```python
from build123d import *

# Parameters (mm, degrees)
EXTRUDE_1_DEPTH     = 50
SKETCH_3_R          = 2.5
CUT_EXTRUDE_1_DEPTH = 74.539294107
SKETCH_4_W          = 29.863739494
SKETCH_4_H          = 8.563866473
EXTRUDE_2_DEPTH     = 37


with BuildPart() as part:
    # 草图2 → 凸台-拉伸1 (new, symmetric)
    with BuildSketch(Plane.XY):
        Polygon((-30, 19.5), (30, 19.5), (30, -16.666666667), (40, -16.666666667), (40, -19.5), (-40, -19.5), (-40, -16.666666667), (-30, -16.666666667), align=None)
    extrude(amount=EXTRUDE_1_DEPTH, both=True)

    # 草图3 → 切除-拉伸1 (cut, through all)
    with BuildSketch(Plane(origin=(0, -16.666666667, 0), x_dir=(1, 0, 0), z_dir=(0, 1, 0))):
        with Locations(Location((-35, 24, 0), (0, 0, 270))):
            Circle(SKETCH_3_R)
        with Locations(Location((35, 24, 0), (0, 0, 270))):
            Circle(SKETCH_3_R)
        with Locations(Location((-35, -24, 0), (0, 0, 270))):
            Circle(SKETCH_3_R)
        with Locations(Location((35, -24, 0), (0, 0, 270))):
            Circle(SKETCH_3_R)
    extrude(amount=-CUT_EXTRUDE_1_DEPTH, mode=Mode.SUBTRACT)

    # 草图4 → 凸台-拉伸2 (add)
    with BuildSketch(Plane.XY.offset(50)):
        with Locations((0, -12.959263215)):
            Rectangle(SKETCH_4_W, SKETCH_4_H)
    extrude(amount=EXTRUDE_2_DEPTH)


solid = part.part
```
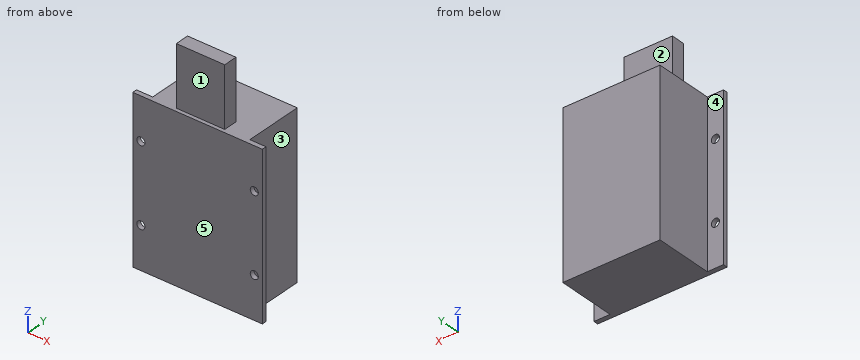
The model under review builds one solid part; all positions refer to its coordinate system, in mm. Face numbers are marked on the shaded views. A direction names the side the tool comes from. Round coordinates to 2 decimals unless told otherwise and drop trailing zeros. Write each loop counter-clockwise with the first axis right and the second up, starting at its lowest first coordinate (ties: lowest second). Pieces come first, ordered by that corner, then holes. Notation, with made-up numbers: M 1,10 L 13,10 A18 cw 13,33 Z; hole C 81.25,-9.5 d9. An arc over 180 degrees is marked long. Use CSV: the item, a comma, the result in double quotes. Start each with the question number.
(1) We need section A-A, the plane z = 24. State the section outline as (x, y) points.
(2) We need section B-B, the plane x = 35. State the section outline as (y, z) points.
(3) For line 1 along X through (y, z) = (-18.3, 24); line 2 along Z through (x, y) = (4, 2.5); line 3 along Y through (x, z) = (-9, 71.5), list the stretches that pass through material, from the lowest coordinate up.
(4) We need section D-D, the plane y = -13. State the section outline as (x, z) points, then the cut area to 3 significant figures.
(5) We need section C-C, the plane z = -4. State the section outline as (x, y) points.
(6) Tool access review of the marked faces 1, 2, 3, 4 and 5: name each direction out of +Z, -Z, +X, -X, +Y, -Y from which nothing blocks a thin tool from reaching the whole face with its end or side.
(7) Clearance check with flat-ended pins moving along their axes: P1, Ø8, axis at x = -7, z = 63.5, coming from the -Y side; P2, Ø2.5, axis at y = -14.5, z = 66, coming from the +X side; P3, Ø18, axis at y = 7, z = -8.5, coming from the -X side. State where each tip first meets the part, or that it passes through.
Findings:
1,outline,"M -40,-19.5 L -37.5,-19.5 L -37.5,-16.67 L -40,-16.67 Z; M -32.5,-19.5 L 32.5,-19.5 L 32.5,-16.67 L 30,-16.67 L 30,19.5 L -30,19.5 L -30,-16.67 L -32.5,-16.67 Z; M 37.5,-19.5 L 40,-19.5 L 40,-16.67 L 37.5,-16.67 Z"
2,outline,"M -19.5,-50 L -16.67,-50 L -16.67,-26.5 L -19.5,-26.5 Z; M -19.5,-21.5 L -16.67,-21.5 L -16.67,21.5 L -19.5,21.5 Z; M -19.5,26.5 L -16.67,26.5 L -16.67,50 L -19.5,50 Z"
3,line 1,"-40 to -37.5, -32.5 to 32.5, 37.5 to 40"
3,line 2,"-50 to 50"
3,line 3,"-17.24 to -8.68"
4,outline,"M -30,-50 L 30,-50 L 30,50 L 14.93,50 L 14.93,87 L -14.93,87 L -14.93,50 L -30,50 Z"
4,area,"7,100 mm^2"
5,outline,"M -40,-19.5 L 40,-19.5 L 40,-16.67 L 30,-16.67 L 30,19.5 L -30,19.5 L -30,-16.67 L -40,-16.67 Z"
6,face 1,"+Z, +X, -X, -Y"
6,face 2,"+Z, +X, -X, +Y"
6,face 3,"+Z, -Z, +X, +Y"
6,face 4,"+Z, -Z, -X, +Y"
6,face 5,"+Z, -Z, +X, -X, -Y"
7,P1,"y = -17.24"
7,P2,"x = 14.93"
7,P3,"x = -30"
